from build123d import *

# Parameters (mm, degrees)
F0_R     = 17
F1_DEPTH = 3
F2_DEPTH = 24


with BuildPart() as f1:
    # F0 (on Top) → F1 (new body)
    with BuildSketch(Plane.XY):
        with BuildLine():
            ThreePointArc((18.966954023, 1.1201138736), (19.9859901049, 2.4265755892), (21.5431034483, 2.9928571327))
            ThreePointArc((21.5431034483, 2.9928571327), (0, 21.75), (-21.5431034483, 2.9928571327))
            ThreePointArc((-21.5431034483, 2.9928571327), (-19.9859901049, 2.4265755892), (-18.966954023, 1.1201138736))
            ThreePointArc((-18.966954023, 1.1201138736), (0, 19), (18.966954023, 1.1201138736))
        make_face()
        with BuildLine():
            ThreePointArc((-21.5431034483, -2.9928571327), (0, -21.75), (21.5431034483, -2.9928571327))
            ThreePointArc((21.5431034483, -2.9928571327), (19.9859901049, -2.4265755892), (18.966954023, -1.1201138736))
            ThreePointArc((18.966954023, -1.1201138736), (0, -19), (-18.966954023, -1.1201138736))
            ThreePointArc((-18.966954023, -1.1201138736), (-19.9859901049, -2.4265755892), (-21.5431034483, -2.9928571327))
        make_face()
        with BuildLine():
            ThreePointArc((18.966954023, -1.1201138736), (18.75, 0), (18.966954023, 1.1201138736))
            ThreePointArc((18.966954023, 1.1201138736), (0, 19), (-18.966954023, 1.1201138736))
            ThreePointArc((-18.966954023, 1.1201138736), (-18.8047378783, 0.5704656295), (-18.75, 0))
            ThreePointArc((-18.75, 0), (-18.8047378783, -0.5704656295), (-18.966954023, -1.1201138736))
            ThreePointArc((-18.966954023, -1.1201138736), (0, -19), (18.966954023, -1.1201138736))
        make_face()
        Circle(F0_R, mode=Mode.SUBTRACT)
    extrude(amount=F1_DEPTH)

    # F0 (on Top) → F2 (join)
    with BuildSketch(Plane.XY):
        with BuildLine():
            ThreePointArc((18.966954023, -1.1201138736), (18.75, 0), (18.966954023, 1.1201138736))
            ThreePointArc((18.966954023, 1.1201138736), (0, 19), (-18.966954023, 1.1201138736))
            ThreePointArc((-18.966954023, 1.1201138736), (-18.8047378783, 0.5704656295), (-18.75, 0))
            ThreePointArc((-18.75, 0), (-18.8047378783, -0.5704656295), (-18.966954023, -1.1201138736))
            ThreePointArc((-18.966954023, -1.1201138736), (0, -19), (18.966954023, -1.1201138736))
        make_face()
        Circle(F0_R, mode=Mode.SUBTRACT)
        with BuildLine():
            ThreePointArc((-18.75, 0), (-18.8047378783, 0.5704656295), (-18.966954023, 1.1201138736))
            ThreePointArc((-18.966954023, 1.1201138736), (-19, 0), (-18.966954023, -1.1201138736))
            ThreePointArc((-18.966954023, -1.1201138736), (-18.8047378783, -0.5704656295), (-18.75, 0))
        make_face()
        with BuildLine():
            ThreePointArc((19, 0), (18.9917367089, 0.5603006172), (18.966954023, 1.1201138736))
            ThreePointArc((18.966954023, 1.1201138736), (18.75, 0), (18.966954023, -1.1201138736))
            ThreePointArc((18.966954023, -1.1201138736), (18.9917367089, -0.5603006172), (19, 0))
        make_face()
    extrude(amount=F2_DEPTH)


solid = f1.part
For this review, take the finished solid that the model builds, in its own axes (mm). A direction names the side the tool comes from. Round coordinates to 2 decimals unless told otherwise and drop trailing zeros. Order: outer loops, then holes, each group sorted by start corner. A loop starts at its lowest first (then second) coordinate and runs counter-clockwise, first axis right, second up. Notation, with made-up numbers: (9, 55) -> (45, 55) arc R24 ccw to (45, 73) -> close; hole circle Ø2 at (4, 58). An arc over 180 degrees is marked (long way). Put each result on its own line as item: value.
Q1. Machinability: for faces 5 (the cylindrical face through (20.005, -2.44, 1.479)), 6 (the flat face through (3, -19, 3)), 7 (the cylindrical face through (-20.005, 2.44, 1.479)), 8 (the flat face through (-14, -10, 24)), which of the approach directions +Z, -Z, +X, -X, +Y, -Y give a long, thin tool a straight path to every point of the face, cutting with its end or side? Answer none if there is none.
Check result:
face 5: +Z, -Z, +X
face 6: +Z, -Y
face 7: +Z, -Z, -X
face 8: +Z, +X, -X, +Y, -Y
Q2. Add section C-C on x = -7. Write out the cut boundary in (y, z).
Check result:
outline: (-20.59, 0) -> (-15.49, 0) -> (-15.49, 24) -> (-17.66, 24) -> (-17.66, 3) -> (-20.59, 3) -> close; (15.49, 0) -> (20.59, 0) -> (20.59, 3) -> (17.66, 3) -> (17.66, 24) -> (15.49, 24) -> close
Q3. For probe 1 along Y at (x, z) = (0, 6.25); probe 2 along Z at (x, y) = (7, 19.5); probe 3 along Y at (x, z) = (-5, 4.75), list the stretches that pass through material, from the lowest coordinate up. Write a range as [from, to].
Check result:
probe 1: [-19, -17], [17, 19]
probe 2: [0, 3]
probe 3: [-18.33, -16.25], [16.25, 18.33]
Q4. Mouldability with a two-part tool opening along Y and no side actions: class faces 1 (the cylindrical face through (-0.436, -21.746, 1.479)), 2 (the cylindrical face through (-19.967, -2.413, 1.479)), 3 (the cylindrical face through (0.436, 21.746, 1.479)), 4 (the flat face through (1.5, 19.1, 3)) as pulls with the +Y half, pulls with the -Y half, needs draft (parallel to the pull), parting line crosses it, or undercut.
Check result:
face 1: pulls with the -Y half
face 2: undercut
face 3: pulls with the +Y half
face 4: needs draft
Q5. Insertion check: pin 1 Ø2 at (y, z) = (14, 13.5) entering from +X; pin 2 Ø8 at (y, z) = (2.5, 10) entering from -X; pin 3 Ø20.5 at (x, y) = (0, 0) entering from +Z; pin 4 Ø4 at (y, z) = (-2.5, 11.5) entering from +X. Each pin has a flat end and moves straight along its axis. Give the tip position at first contact, or say it passes through.
Check result:
pin 1: x = 13.86
pin 2: x = -19
pin 3: through
pin 4: x = 18.99
Q6. Add section A-A on x = 0. Write out the cut boundary in (y, z), plus the area to 4 significant figures.
Check result:
outline: (-21.75, 0) -> (-17, 0) -> (-17, 24) -> (-19, 24) -> (-19, 3) -> (-21.75, 3) -> close; (17, 0) -> (21.75, 0) -> (21.75, 3) -> (19, 3) -> (19, 24) -> (17, 24) -> close
area: 112.5 mm2
Q7. Add section B-B on z = 20.5. Write out the cut boundary in (x, y), plus the area to 3 significant figures.
Check result:
outline: circle Ø38 at (0, 0); hole circle Ø34 at (0, 0)
area: 226 mm2
